The listing builds one solid part. Answer for the finished solid, in the listing's coordinates (mm). Face numbers are marked on the shaded views. A direction names the side the tool comes from. Coordinates: 2 decimals unless noted, no trailing zeros. Order: outer loops, then holes, each group sorted by start corner. A loop starts at its lowest first (then second) coordinate and runs counter-clockwise, first axis right, second up. Notation, with made-up numbers: (63, 33.25) -> (88, 33.25) arc R21 ccw to (88, 48.25) -> close; hole circle Ø8 at (-15.75, 37). An arc over 180 degrees is marked (long way). Return JSON: item names as keys, results as strings.
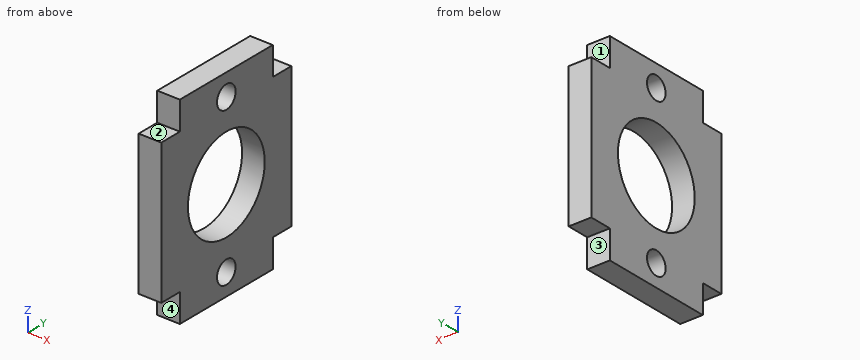
from build123d import *

# Parameters (mm, degrees)
SKETCH1_R           = 10.499999955
SKETCH1_R_2         = 2.54
BOSS_EXTRUDE1_DEPTH = 5.08


with BuildPart() as part:
    # Sketch1 → Boss-Extrude1 (new body)
    with BuildSketch(Plane(origin=(0, 0, 0), x_dir=(0, 0, -1), z_dir=(1, 0, 0))):
        Polygon((-22.225, 12.7), (-15.875, 12.7), (-15.875, 17.78), (15.875, 17.78), (15.875, 12.7), (22.225, 12.7), (22.225, -12.7), (15.875, -12.7), (15.875, -17.78), (-15.875, -17.78), (-15.875, -12.7), (-22.225, -12.7), align=None)
        Circle(SKETCH1_R, mode=Mode.SUBTRACT)
        with Locations((-17.346281091, 0)):
            Circle(SKETCH1_R_2, mode=Mode.SUBTRACT)
        with Locations((17.346281091, 0)):
            Circle(SKETCH1_R_2, mode=Mode.SUBTRACT)
    extrude(amount=BOSS_EXTRUDE1_DEPTH)


solid = part.part
1. The part is cut by section C-C on y = -4.5. Give the vertices of the cut face in (x, z) (3 decimals).
Answer block:
{"outline": "(0, -22.225) -> (5.08, -22.225) -> (5.08, -9.487) -> (0, -9.487) -> close; (0, 9.487) -> (5.08, 9.487) -> (5.08, 22.225) -> (0, 22.225) -> close"}
2. Consider line 1 (Z direction, x = 0.35, y = -1) (3 decimals); line 2 (Y direction, x = 1.2, z = 0); line 3 (Z direction, x = 4.25, y = -13.5) (3 decimals). Determine where each line is inside the solid, lowest interval first. Write a range as from..to.
Answer block:
{"line 1": "z = -22.225..-19.681, -15.011..-10.452, 10.452..15.011, 19.681..22.225", "line 2": "y = -17.78..-10.5, 10.5..17.78", "line 3": "z = -15.875..15.875"}
3. For the marked faces 1, 2, 3 and 4, determine the directions among +Z, -Z, +X, -X, +Y, -Y from which every point of the face is accessible in a straight line to the end or side of a thin tool.
Answer block:
{"face 1": "+Z, +X, -X, +Y", "face 2": "+Z, +X, -X, -Y", "face 3": "-Z, +X, -X, +Y", "face 4": "-Z, +X, -X, -Y"}
4. Each of these flat-tipped pins is pushed along its axis until it touches: pin 1 Ø2.5 at (x, y) = (3.5, 14.5) entering from +Z (3 decimals); pin 2 Ø2 at (y, z) = (9.5, -5) entering from -X; pin 3 Ø1.5 at (x, z) = (3.5, 20) entering from -Y; pin 4 Ø1.5 at (x, y) = (1.5, -15) entering from -Z (3 decimals). Where does it stop, or does it pass through?
Answer block:
{"pin 1": "stops at z = 15.875", "pin 2": "stops at x = 0", "pin 3": "stops at y = -12.7", "pin 4": "stops at z = -15.875"}
5. The part is cut by section A-A on y = 0. Give the vertices of the cut face in (x, z) (3 decimals).
Answer block:
{"outline": "(0, -22.225) -> (5.08, -22.225) -> (5.08, -19.886) -> (0, -19.886) -> close; (0, -14.806) -> (5.08, -14.806) -> (5.08, -10.5) -> (0, -10.5) -> close; (0, 10.5) -> (5.08, 10.5) -> (5.08, 14.806) -> (0, 14.806) -> close; (0, 19.886) -> (5.08, 19.886) -> (5.08, 22.225) -> (0, 22.225) -> close"}
6. The part is cut by section D-D on y = -14. Give the vertices of the cut face in (x, z) (3 decimals).
Answer block:
{"outline": "(0, -15.875) -> (5.08, -15.875) -> (5.08, 15.875) -> (0, 15.875) -> close"}
7. The part is cut by section B-B on z = 0. Give the vertices of the cut face in (x, y), and give its area (3 significant figures).
Answer block:
{"outline": "(0, -17.78) -> (5.08, -17.78) -> (5.08, -10.5) -> (0, -10.5) -> close; (0, 10.5) -> (5.08, 10.5) -> (5.08, 17.78) -> (0, 17.78) -> close", "area": "74.0 mm2"}
